from build123d import *

# Parameters (mm, degrees)
F0_W     = 50
F0_H     = 200
F1_DEPTH = 2150
F4_DEPTH = 50
F6_DEPTH = 50


with BuildPart() as f1:
    # F0 (on Front) → F1 (new body)
    with BuildSketch(Plane.XZ):
        Rectangle(F0_W, F0_H)
    extrude(amount=F1_DEPTH)

    # F3 (on face) → F4 (cut)
    with BuildSketch(Plane.YZ.offset(25)):
        Polygon((-1900, -100), (-1900, -55.918255), (-2150, -100), align=None)
    extrude(amount=-F4_DEPTH, mode=Mode.SUBTRACT)

    # F5 (on face) → F6 (cut)
    with BuildSketch(Plane.YZ.offset(25)):
        Polygon((-250, -55.918255), (-250, -100), (0, -100), align=None)
    extrude(amount=-F6_DEPTH, mode=Mode.SUBTRACT)


solid = f1.part
For this review, take the finished solid that the model builds, in its own axes (mm). A direction names the side the tool comes from. Coordinates: 2 decimals unless noted, no trailing zeros. Loops run counter-clockwise (first coordinate to the right, second up) from the corner with the lowest first, then second, coordinate; pieces in that order, holes last. Notation, with made-up numbers: (-1, -6.5) - (10, -6.5) arc R27 cw to (10, 24.5) - close; hole circle Ø11 at (-31.5, 88). An arc over 180 degrees is marked (long way). Return JSON: item names as keys, results as strings.
Item 1: For line 1 (Z direction, x = -13.5, y = -97.5); line 2 (Z direction, x = -4.5, y = -215), list the stretches that pass through material, from the lowest coordinate up.
Determined:
{"line 1": "z = -82.81 to 100", "line 2": "z = -62.09 to 100"}
Item 2: For faces 5 (the flat face through (0, -250, -78)), 6 (the flat face through (-25, -1060, -1)), list the 3-axis set-ups (+Z, -Z, +X, -X, +Y, -Y) from which the entire face can be reached by the end or side of a thin tool; tool diameter is ignored.
Determined:
{"face 5": "-Z, +X, -X", "face 6": "+Z, -Z, -X, +Y, -Y"}
Item 3: Mouldability with a two-part tool opening along Y and no side actions: class faces 1 (the flat face through (0, -1900, -78)), 2 (the flat face through (0, -2150, 1)), 3 (the flat face through (0.35, -2023.25, -77.65)), 4 (the flat face through (0, -1063, -100)) as pulls with the +Y half, pulls with the -Y half, needs draft (parallel to the pull), parting line crosses it, or undercut.
Determined:
{"face 1": "undercut", "face 2": "pulls with the -Y half", "face 3": "undercut", "face 4": "needs draft"}
Item 4: Take a section at A-A (x = 3.5). Give the boundary of the cut face in (y, z).
Determined:
{"outline": "(-2150, -100) - (-1900, -55.92) - (-1900, -100) - (-250, -100) - (-250, -55.92) - (0, -100) - (0, 100) - (-2150, 100) - close"}
Item 5: Take a section at B-B (y = -186). Give the boundary of the cut face in (x, z), then the cut area to 3 significant figures.
Determined:
{"outline": "(-25, -67.2) - (25, -67.2) - (25, 100) - (-25, 100) - close", "area": "8,360 mm2"}
